from build123d import *

# Parameters (mm, degrees)
ESQUISSE1_W             = 29.5
ESQUISSE1_H             = 13.8
ESQUISSE1_R             = 1.6
BOSS_EXTRU_1_DEPTH      = 6
ESQUISSE2_R             = 2.35
ENL_V_MAT_EXTRU_1_DEPTH = 7
ESQUISSE3_R             = 3.75
ENL_V_MAT_EXTRU_2_DEPTH = 4
ESQUISSE5_W             = 5
ESQUISSE5_H             = 8
ENL_V_MAT_EXTRU_3_DEPTH = 3


with BuildPart() as part:
    # Esquisse1 → Boss.-Extru.1 (new body)
    with BuildSketch(Plane(origin=(0, 0, 0), x_dir=(1, 0, 0), z_dir=(0, 1, 0))):
        with Locations((14.75, 6.9)):
            Rectangle(ESQUISSE1_W, ESQUISSE1_H)
        with Locations((25, 6.9)):
            Circle(ESQUISSE1_R, mode=Mode.SUBTRACT)
    extrude(amount=BOSS_EXTRU_1_DEPTH)

    # Esquisse2 → Enlèv. mat.-Extru.1 (cut, through all)
    with BuildSketch(Plane(origin=(0, 6, 0), x_dir=(1, 0, 0), z_dir=(0, 1, 0))):
        with Locations((0, 6.9)):
            Circle(ESQUISSE2_R)
    extrude(amount=-ENL_V_MAT_EXTRU_1_DEPTH, mode=Mode.SUBTRACT)

    # Esquisse3 → Enlèv. mat.-Extru.2 (cut)
    with BuildSketch(Plane(origin=(0, 6, 0), x_dir=(1, 0, 0), z_dir=(0, 1, 0))):
        with Locations((0, 6.9)):
            Circle(ESQUISSE3_R)
    extrude(amount=-ENL_V_MAT_EXTRU_2_DEPTH, mode=Mode.SUBTRACT)

    # Symétrie1: part across plane


with BuildPart() as part_1:
    add(part.part)
    add(part.part.mirror(Plane(origin=(0, 6, 0), x_dir=(0, 0, 1), z_dir=(1, 0, 0))))

    # Esquisse5 → Enlèv. mat.-Extru.3 (cut)
    with BuildSketch(Plane.XZ.offset(-6)):
        with Locations((18.1, -6.9)):
            Rectangle(ESQUISSE5_W, ESQUISSE5_H)
    extrude(amount=ENL_V_MAT_EXTRU_3_DEPTH, mode=Mode.SUBTRACT)


solid = part_1.part
Input: part model. Units: mm. Frame: model coordinates. A direction names the side the tool comes from. Give positions to 0.01 mm unless a question says otherwise; leave off trailing zeros. Order: outer loops, then holes, each group sorted by start corner. A loop starts at its lowest first (then second) coordinate and runs counter-clockwise, first axis right, second up. Notation, with made-up numbers: (80.5, 49) - (117.5, 49) arc R20 ccw to (117.5, 82) - close; hole circle Ø11 at (-28.5, -20.5). An arc over 180 degrees is marked (long way). Write each question's results on one line, items separated by ' | '.
Item 1: Section C-C (y = 5). Return loops of the section in (x, z), and give its area (3 significant figures).
A:
outline: (-29.5, -13.8) - (29.5, -13.8) - (29.5, 0) - (-29.5, 0) - close; hole circle Ø3.2 at (-25, -6.9); hole circle Ø7.5 at (0, -6.9); hole (15.6, -10.9) - (20.6, -10.9) - (20.6, -2.9) - (15.6, -2.9) - close; hole circle Ø3.2 at (25, -6.9) | area: 714 mm^2
Item 2: Access query for faces 1 (the flat face through (0, 0, -4)), 2 (the flat face through (18, 5, -10.9)). Directions: +Z, -Z, +X, -X, +Y, -Y. A direction counts if a zero-diameter tool reaches every point of the face in a straight line with its end or side. Return the directions, or none.
A:
face 1: +Z, -Z, +X, -X, -Y | face 2: +Y
Item 3: Contact query for flat-ended pins moving along their axis: pin 1 Ø1.9 at (x, z) = (25, -6.9) entering from -Y; pin 2 Ø1.9 at (x, z) = (1.5, -7) entering from +Y; pin 3 Ø1 at (x, z) = (-3, -10.5) entering from -Y. Output: stop coordinate, or through.
A:
pin 1: passes through | pin 2: stops at y = 2 | pin 3: stops at y = 0
Item 4: Draft query along X for faces 3 (the cylindrical face through (-23.82, 2.96, -7.98)), 4 (the flat face through (29.5, 3, -7)), 5 (the flat face through (0, 3, -13.8)). Return one class per face: released by +X, released by -X, zero draft, split by the parting line, or undercut.
A:
face 3: undercut | face 4: released by +X | face 5: zero draft
Item 5: Material intervals for line 1 along X through (y, z) = (1.5, -6.9); line 2 along X through (y, z) = (2.75, -6.9); line 3 along X through (y, z) = (4.85, -6.9), sorted ascending.
A:
line 1: x = -29.5 to -26.6, -23.4 to -2.35, 2.35 to 23.4, 26.6 to 29.5 | line 2: x = -29.5 to -26.6, -23.4 to -3.75, 3.75 to 23.4, 26.6 to 29.5 | line 3: x = -29.5 to -26.6, -23.4 to -3.75, 3.75 to 15.6, 20.6 to 23.4, 26.6 to 29.5
Item 6: Section B-B (z = -6.9). Return loops of the section in (x, y).
A:
outline: (-29.5, 0) - (-26.6, 0) - (-26.6, 6) - (-29.5, 6) - close; (-23.4, 0) - (-2.35, 0) - (-2.35, 2) - (-3.75, 2) - (-3.75, 6) - (-23.4, 6) - close; (2.35, 0) - (23.4, 0) - (23.4, 6) - (20.6, 6) - (20.6, 3) - (15.6, 3) - (15.6, 6) - (3.75, 6) - (3.75, 2) - (2.35, 2) - close; (26.6, 0) - (29.5, 0) - (29.5, 6) - (26.6, 6) - close
Item 7: Section A-A (x = 25). Return loops of the section in (y, z).
A:
outline: (0, -13.8) - (6, -13.8) - (6, -8.5) - (0, -8.5) - close; (0, -5.3) - (6, -5.3) - (6, 0) - (0, 0) - close
